Part print with two shaded views. Sizes in mm from the minimum x, y, z corner. A direction names the side the tool comes from. Round coordinates to 2 decimals unless told otherwise and drop trailing zeros. Write each loop counter-clockwise with the first axis right and the second up, starting at its lowest first coordinate (ties: lowest second). Pieces come first, ordered by that corner, then holes. Notation, with made-up numbers: (47, 43.5) -> (56, 43.5) arc R21 cw to (56, 66.5) -> close; hole circle Ø8 at (75.5, 56). An arc over 180 degrees is marked (long way). Return JSON: item names as keys, results as strings.
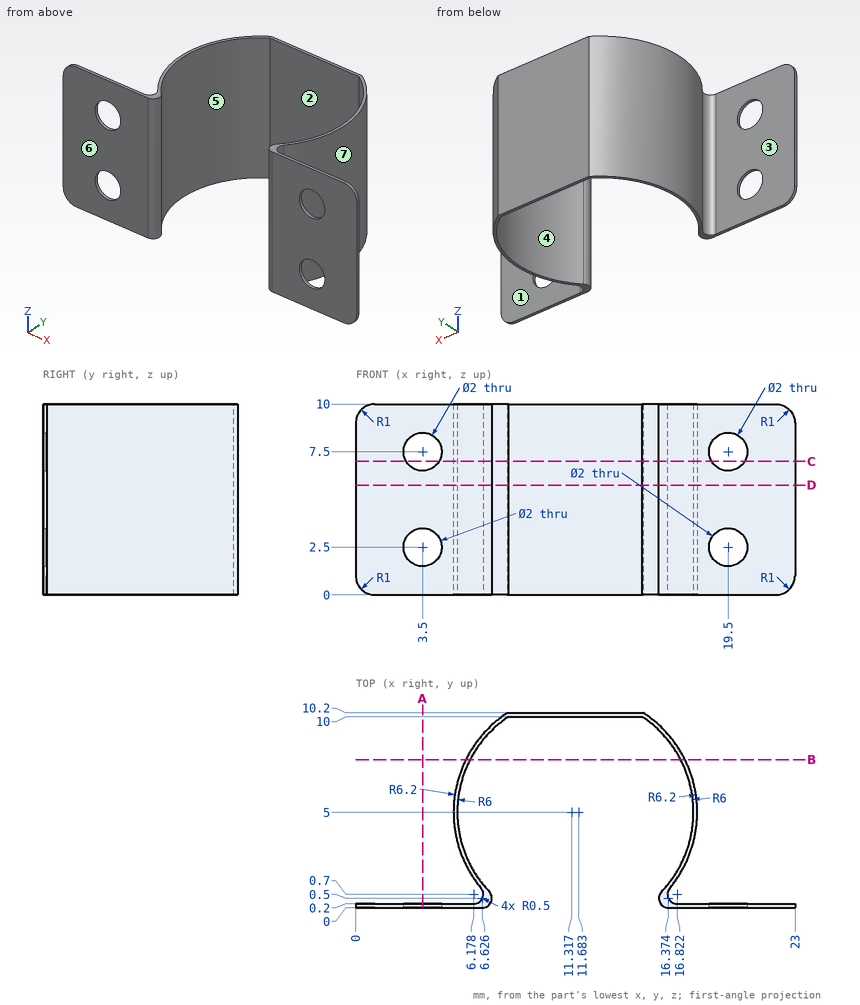
Q1. Saw through at D-D on z = 5.75. List the corners of the cut face in (x, y).
Verdict:
{"outline": "(0, 0) -> (6.63, 0) arc R0.5 ccw to (6.99, 0.85) arc R6 cw to (8, 10) -> (15, 10) arc R6 cw to (16.01, 0.85) arc R0.5 ccw to (16.37, 0) -> (23, 0) -> (23, 0.2) -> (16.82, 0.2) arc R0.5 cw to (16.44, 1.02) arc R6.2 ccw to (15.06, 10.2) -> (7.94, 10.2) arc R6.2 ccw to (6.56, 1.02) arc R0.5 cw to (6.18, 0.2) -> (0, 0.2) -> close"}
Q2. Saw through at A-A on x = 3.5. List the corners of the cut face in (y, z).
Verdict:
{"outline": "(0, 0) -> (0.2, 0) -> (0.2, 1.5) -> (0, 1.5) -> close; (0, 3.5) -> (0.2, 3.5) -> (0.2, 6.5) -> (0, 6.5) -> close; (0, 8.5) -> (0.2, 8.5) -> (0.2, 10) -> (0, 10) -> close"}
Q3. Wall check: L1, parallel to Z at x = 3.5, y = 0.15; L2, parallel to X at y = 0.15, z = 2.5 (1 decimal); L3, parallel to Y at x = 16.75, z = 4 (1 decimal). Give the ranges that are in metal, low to high.
Verdict:
{"L1": "z = 0 to 1.5, 3.5 to 6.5, 8.5 to 10", "L2": "x = 0 to 2.5, 4.5 to 7, 16 to 18.5, 20.5 to 23", "L3": "y = 0 to 0.2, 1.4 to 1.8, 8.2 to 8.6"}
Q4. Two-plate mould, pull along X, no slides. Class the marked faces 5, 6 and 7: +X half, -X half, draft (parallel to the pull), parting line (faces both ways), or undercut.
Verdict:
{"face 5": "undercut", "face 6": "draft", "face 7": "+X half"}
Q5. 3-axis set-ups, long thin cutter, end or side, ignore diameter. For the marked faces 1, 2, 3 and 4: which of +Z, -Z, +X, -X, +Y, -Y reach the whole face in a straight line?
Verdict:
{"face 1": "+Z, -Z, +X", "face 2": "+Z, -Z, -Y", "face 3": "+Z, -Z, -X", "face 4": "+Z, -Z"}
Q6. Saw through at C-C on z = 7. List the corners of the cut face in (x, y).
Verdict:
{"outline": "(0, 0) -> (2.63, 0) -> (2.63, 0.2) -> (0, 0.2) -> close; (4.37, 0) -> (6.63, 0) arc R0.5 ccw to (6.99, 0.85) arc R6 cw to (8, 10) -> (15, 10) arc R6 cw to (16.01, 0.85) arc R0.5 ccw to (16.37, 0) -> (18.63, 0) -> (18.63, 0.2) -> (16.82, 0.2) arc R0.5 cw to (16.44, 1.02) arc R6.2 ccw to (15.06, 10.2) -> (7.94, 10.2) arc R6.2 ccw to (6.56, 1.02) arc R0.5 cw to (6.18, 0.2) -> (4.37, 0.2) -> close; (20.37, 0) -> (23, 0) -> (23, 0.2) -> (20.37, 0.2) -> close"}
Q7. Pin check, flat tips, straight feed: pin 1 Ø2.5 at (x, z) = (3.5, 2.5) entering from +Y; pin 2 Ø1.8 at (x, z) = (3.5, 7.5) entering from +Y; pin 3 Ø5.5 at (x, z) = (12.5, 3) entering from -Y (1 decimal); pin 4 Ø5 at (x, z) = (19, 9) entering from +Y (1 decimal). Stop position of each tip, or through.
Verdict:
{"pin 1": "stops at y = 0.2", "pin 2": "passes through", "pin 3": "stops at y = 9.8", "pin 4": "stops at y = 8.9"}
Q8. Saw through at B-B on y = 7.75. List the corners of the cut face in (x, z).
Verdict:
{"outline": "(5.76, 0) -> (5.98, 0) -> (5.98, 10) -> (5.76, 10) -> close; (17.02, 0) -> (17.24, 0) -> (17.24, 10) -> (17.02, 10) -> close"}
